from build123d import *

# Parameters (mm, degrees)
BASE_DEPTH  = 2.286
WALLS_DEPTH = 36.1315


with BuildPart() as part:
    # Sketch1 → Base (new body)
    with BuildSketch(Plane(origin=(0, 0, 0), x_dir=(1, 0, 0), z_dir=(0, 1, 0))):
        Polygon((-46.99, 0), (46.99, 0), (25.26665, -132.4864), (-25.26665, -132.4864), align=None)
        with BuildLine():
            Line((-11.1633, -8.773780407), (-3.233109796, -8.773780407))
            ThreePointArc((-3.233109796, -8.773780407), (0, -5.540670611), (3.233109796, -8.773780407))
            Line((3.233109796, -8.773780407), (11.1633, -8.773780407))
            ThreePointArc((11.1633, -8.773780407), (14.396409796, -12.006890204), (11.1633, -15.24))
            Line((11.1633, -15.24), (-11.1633, -15.24))
            ThreePointArc((-11.1633, -15.24), (-14.396409796, -12.006890204), (-11.1633, -8.773780407))
        make_face(mode=Mode.SUBTRACT)
    extrude(amount=BASE_DEPTH)

    # Sketch1_4 → Walls (add)
    with BuildSketch(Plane(origin=(0, 0, 0), x_dir=(1, 0, 0), z_dir=(0, 1, 0))):
        Polygon((-25.26665, -132.4864), (25.26665, -132.4864), (46.99, 0), (43.999607163, -2.54), (23.1092077, -129.9464), (-23.1092077, -129.9464), (-43.999607163, -2.54), (-46.99, 0), align=None)
    extrude(amount=WALLS_DEPTH)


solid = part.part
Can you work these out from the model? Positions are in its coordinate system, mm. A direction names the side the tool comes from. Give positions to 0.01 mm unless a question says otherwise; leave off trailing zeros. Loops run counter-clockwise (first coordinate to the right, second up) from the corner with the lowest first, then second, coordinate; pieces in that order, holes last. Notation, with made-up numbers: (52, 38) - (67, 38) arc R17 cw to (67, 53) - close; hole circle Ø6 at (-23.5, 72.5). An arc over 180 degrees is marked (long way). Answer as a JSON object with one key per item and string values.
Q1. If I drill on L1, parallel to Z at x = 11.5, y = 2; L2, parallel to Y at x = -25, z = 16.5; L3, parallel to X at y = 17.5, z = 103.5, over which ranges is the centre line in solid material (lowest first)?
Geometry says:
{"L1": "0 to 8.79, 15.22 to 132.49", "L2": "0 to 2.29", "L3": "-30.02 to -27.45, 27.45 to 30.02"}
Q2. Will these pins go through, and if not, where does the flat tip stop? P1, Ø3, axis at y = 19.5, z = 96.5, coming from the -X side; P2, Ø6, axis at x = 4, y = 31, coming from the -Z side; P3, Ø5, axis at y = 10.5, z = 95, coming from the +X side.
Geometry says:
{"P1": "x = -31.41", "P2": "z = 129.95", "P3": "x = 31.82"}
Q3. Imagine slicing it at C-C on z = 122. Write out the boundary of the cut face in (x, y), plus the area to 3 significant figures.
Geometry says:
{"outline": "(-26.99, 0) - (26.99, 0) - (26.99, 36.13) - (24.41, 36.13) - (24.41, 2.29) - (-24.41, 2.29) - (-24.41, 36.13) - (-26.99, 36.13) - close", "area": "298 mm²"}
Q4. Imagine slicing it at B-B on y = 5. Write out the boundary of the cut face in (x, z), plus the area to 3 significant figures.
Geometry says:
{"outline": "(-46.99, 0) - (-44, 2.54) - (-23.11, 129.95) - (23.11, 129.95) - (44, 2.54) - (46.99, 0) - (25.27, 132.49) - (-25.27, 132.49) - close", "area": "792 mm²"}
Q5. Imagine slicing it at A-A on x = 0. Write out the boundary of the cut face in (y, z), plus the area to 3 significant figures.
Geometry says:
{"outline": "(0, 0) - (2.29, 0) - (2.29, 5.54) - (0, 5.54) - close; (0, 15.24) - (2.29, 15.24) - (2.29, 129.95) - (36.13, 129.95) - (36.13, 132.49) - (0, 132.49) - close", "area": "367 mm²"}
Q6. Imagine slicing it at D-D on x = -17.5. Write out the boundary of the cut face in (y, z), plus the area to 3 significant figures.
Geometry says:
{"outline": "(0, 0) - (2.29, 0) - (2.29, 129.95) - (36.13, 129.95) - (36.13, 132.49) - (0, 132.49) - close", "area": "389 mm²"}
Q7. If we mould it in two halves opening along X, with no side actions, what happens to faces 4 (the flat face through (-33.408, 18.972, 67.135)), 5 (the flat face through (-35.976, 17.813, 67.171)), 6 (the flat face through (-32, 36.132, 81)), 7 (the cylindrical face through (-14.396, 1.127, 12.078))? For each: pulls with the +X half, pulls with the -X half, needs draft (parallel to the pull), parting line crosses it, or undercut.
Geometry says:
{"face 4": "undercut", "face 5": "pulls with the -X half", "face 6": "needs draft", "face 7": "undercut"}
Q8. Which directions (+Z, -Z, +X, -X, +Y, -Y) give clear straight access to the entire face, cutting with the end or side of a thin tool? Please do faces 1 (the flat face through (1, 0, 65)), 2 (the cylindrical face through (14.396, 1.127, 11.936)), 3 (the flat face through (33.7, 18.97, 65.35)).
Geometry says:
{"face 1": "+Z, -Z, +X, -X, -Y", "face 2": "+Y, -Y", "face 3": "-Z, +Y"}
